Can you work these out from the model? Positions are in its coordinate system, mm. A direction names the side the tool comes from. Round coordinates to 2 decimals unless told otherwise and drop trailing zeros. Write each loop counter-clockwise with the first axis right and the second up, starting at its lowest first coordinate (ties: lowest second). Pieces come first, ordered by that corner, then holes.
Q1. For faces 5 (the flat face through (-12, -53, 42.5)), 6 (the flat face through (-12, -53, 47.5)), 7 (the flat face through (-4, -47, 0)), which set-ups out of +Z, -Z, +X, -X, +Y, -Y let a thin tool reach every point of the face, with its end or its side?
Q2. If we section it at D-D (y = -52.5): Please give me the cut outline in (x, z), plus the area to 3 significant figures.
Q3. If we section it at A-A (z = 45): Please give me the cut outline in (x, y).
Q4. If we section it at C-C (z = 26.5): Please give me the cut outline in (x, y), plus the area to 3 significant figures.
Q5. I'm going to push flat-ended pins straight in: pin 1 Ø2.5 at (y, z) = (-63.5, -51) entering from +X; pin 2 Ø1 at (y, z) = (-57, 32) entering from -X; pin 3 Ø6.5 at (x, z) = (-62, -91) entering from -Y; pin 4 Ø12.5 at (x, y) = (-20.5, -47) entering from -Z. Where does each tip first touch, or does it pass through?
Q6. If we section it at B-B (y = -10.25): Please give me the cut outline in (x, z), plus the area to 3 significant figures.
Q7. We'd pull the mould along Z, two halves only. Please class faces 1 (the flat face through (-17.906, -47.45, 45.035)), 2 (the flat face through (-5, -30, 30)), 3 (the flat face through (-3, -47, 60)), 4 (the cylindrical face through (-68.99, -62.46, -98.15)): +Z half, -Z half, draft (parallel to the pull), parting line (faces both ways), or undercut.
Q8. Please list where these lines run through material, in increasing order: line 1 along Z through (x, y) = (-2.35, -10.25); line 2 along X through (y, z) = (-63.9, -91) (3 decimals); line 3 along Y through (x, z) = (-38, 42.5).
from build123d import *

# Parameters (mm, degrees)
BOSS_EXTRUDE1_DEPTH = 60
SKETCH3_W           = 60
SKETCH3_H           = 5
BOSS_EXTRUDE2_DEPTH = 67
SKETCH4_W           = 20
SKETCH4_H           = 5
BOSS_EXTRUDE3_DEPTH = 101
CUT_EXTRUDE1_REACH  = 139.786
SKETCH6_R           = 5.375
CUT_EXTRUDE2_REACH  = 139.532
SKETCH11_R          = 3.3
FILLET1_R           = 10
FILLET3_R           = 10
FILLET4_R           = 10
BOSS_EXTRUDE4_DEPTH = 2.5


with BuildPart() as part:
    # Sketch1 → Boss-Extrude1 (new body)
    with BuildSketch(Plane.XY):
        Polygon((-5, 0), (-5, -50), (-5, -65), (0, -65), (0, 0), align=None)
    extrude(amount=BOSS_EXTRUDE1_DEPTH)

    # Sketch3 → Boss-Extrude2 (add)
    with BuildSketch(Plane.ZY.offset(5)):
        with Locations((30, -62.5)):
            Rectangle(SKETCH3_W, SKETCH3_H)
    extrude(amount=BOSS_EXTRUDE2_DEPTH)

    # Sketch4 → Boss-Extrude3 (add)
    with BuildSketch(Plane(origin=(0, 0, 0), x_dir=(-1, 0, 0), z_dir=(0, 0, -1))):
        with Locations((62, -62.5)):
            Rectangle(SKETCH4_W, SKETCH4_H)
    extrude(amount=BOSS_EXTRUDE3_DEPTH)

    # Sketch6 → Cut-Extrude1 (cut, up to next)
    with BuildSketch(Plane(origin=(0, -60, 0), x_dir=(1, 0, 0), z_dir=(0, 1, 0)), mode=Mode.PRIVATE) as cut_extrude1_sk1:
        with Locations(Location((-62, 91, 0), (0, 0, 270))):
            Circle(SKETCH6_R)
    cut_extrude1_tool1 = extrude(cut_extrude1_sk1.sketch, amount=-CUT_EXTRUDE1_REACH, mode=Mode.PRIVATE) & part.part
    add(cut_extrude1_tool1.solids().sort_by_distance((-62, -60, -91))[0], mode=Mode.SUBTRACT)

    # Sketch11 → Cut-Extrude2 (cut, up to next)
    with BuildSketch(Plane.ZY.offset(5), mode=Mode.PRIVATE) as cut_extrude2_sk1:
        with Locations(Location((15, -10.25, 0), (0, 0, 270))):
            Circle(SKETCH11_R)
    cut_extrude2_tool1 = extrude(cut_extrude2_sk1.sketch, amount=-CUT_EXTRUDE2_REACH, mode=Mode.PRIVATE) & part.part
    # Sketch11 → Cut-Extrude2 (cut, up to next)
    with BuildSketch(Plane.ZY.offset(5), mode=Mode.PRIVATE) as cut_extrude2_sk2:
        with Locations(Location((45, -10.25, 0), (0, 0, 270))):
            Circle(SKETCH11_R)
    cut_extrude2_tool2 = extrude(cut_extrude2_sk2.sketch, amount=-CUT_EXTRUDE2_REACH, mode=Mode.PRIVATE) & part.part
    add(cut_extrude2_tool1.solids().sort_by_distance((-5, -10.25, 15))[0], mode=Mode.SUBTRACT)
    add(cut_extrude2_tool2.solids().sort_by_distance((-5, -10.25, 45))[0], mode=Mode.SUBTRACT)

    # Fillet1
    fillet1_edges = [part.edges().sort_by_distance(p)[0] for p in [
        (-52, -62.5, -101),
        (-72, -62.5, -101),
    ]]
    fillet(fillet1_edges, radius=FILLET1_R - 0.0001)  # a hair under: the kernel refuses the full size

    # Fillet3
    fillet3_edges = [part.edges().sort_by_distance(p)[0] for p in [
        (-52, -62.5, 0),
    ]]
    fillet(fillet3_edges, radius=FILLET3_R)

    # Fillet4
    fillet4_edges = [part.edges().sort_by_distance(p)[0] for p in [
        (-72, -62.5, 60),
    ]]
    fillet(fillet4_edges, radius=FILLET4_R)

    # Sketch13 → Boss-Extrude4 (add, symmetric)
    with BuildSketch(Plane.XY.offset(45)):
        Polygon((-30.455844123, -60), (-5, -34.544155877), (-5, -60), align=None)
    boss_extrude4 = extrude(amount=BOSS_EXTRUDE4_DEPTH, both=True)

    # Mirror1: Boss-Extrude4 across plane
    add(boss_extrude4.mirror(Plane.XY.offset(30)))


solid = part.part
A:
1. face 5: -X, +Y
1. face 6: +Z, -X, +Y
1. face 7: -Z, +X, +Y, -Y
2. outline: (-22.96, 12.5) - (-5, 12.5) - (-5, 0) - (0, 0) - (0, 60) - (-5, 60) - (-5, 47.5) - (-22.96, 47.5) - (-22.96, 42.5) - (-5, 42.5) - (-5, 17.5) - (-22.96, 17.5) - close
2. area: 480 mm2
3. outline: (-72, -65) - (0, -65) - (0, -13.55) - (-5, -13.55) - (-5, -34.54) - (-30.46, -60) - (-72, -60) - close; (-5, -6.95) - (0, -6.95) - (0, 0) - (-5, 0) - close
4. outline: (-72, -65) - (0, -65) - (0, 0) - (-5, 0) - (-5, -60) - (-72, -60) - close
4. area: 660 mm2
5. pin 1: stops at x = -52
5. pin 2: stops at x = -5
5. pin 3: passes through
5. pin 4: stops at z = 12.5
6. outline: (-5, 0) - (0, 0) - (0, 11.7) - (-5, 11.7) - close; (-5, 18.3) - (0, 18.3) - (0, 41.7) - (-5, 41.7) - close; (-5, 48.3) - (0, 48.3) - (0, 60) - (-5, 60) - close
6. area: 234 mm2
7. face 1: draft
7. face 2: undercut
7. face 3: +Z half
7. face 4: -Z half
8. line 1: z = 0 to 11.7, 18.3 to 41.7, 48.3 to 60
8. line 2: x = -72 to -67.375, -56.625 to -52
8. line 3: y = -65 to -60
